Source: three-view drawing plus pictorial views. Frame: mm from the lowest corner of the part. A direction names the side the tool comes from. Round coordinates to 2 decimals unless told otherwise and drop trailing zeros. Order: outer loops, then holes, each group sorted by start corner. A loop starts at its lowest first (then second) coordinate and runs counter-clockwise, first axis right, second up. Notation, with made-up numbers: (-29.5, -19.75) -> (19.5, -19.75) arc R6 ccw to (19.5, -14.75) -> close; hole circle Ø10 at (4.5, 64). An arc over 180 degrees is marked (long way). Answer as CSV lines item,"result". Start each with the question number.
1) First-contact query: P1, Ø0.6, axis at x = 15, y = 22, coming from the -Z side; P2, Ø12, axis at x = 16, z = 18.5, coming from the +Y side; P3, Ø7, axis at x = 47.5, y = 18.5, coming from the +Z side. Flat tips, straight axial feed; report the tip coordinate or a pass-through.
2) Access query for the marked faces 4 and 5. Directions: +Z, -Z, +X, -X, +Y, -Y. A direction counts if a zero-diameter tool reaches every point of the face in a straight line with its end or side. Return the directions, or none.
3) Section query B-B, the plane x = 14.5. Output: boundary loops of the cut face in (y, z).
4) Mould query, pull axis Z, two halves, no side actions, for the marked faces 1, 2 and 3. Classes: +Z half, -Z half, draft (parallel to the pull), parting line (faces both ways), or undercut.
5) Section query C-C, the plane y = 4. Output: boundary loops of the cut face in (x, z), and give its area (3 significant figures).
6) Section query A-A, the plane z = 33. Output: boundary loops of the cut face in (x, y), and give its area (3 significant figures).
7) Section query D-D, the plane z = 40.5. Output: boundary loops of the cut face in (x, y).
8) Line query: L1, parallel to Y at x = 33, z = 39.5; L2, parallel to Z at x = 34.5, y = 11.5; L3, parallel to Y at x = 17, z = 25. Output: solid intervals per line, ascending.
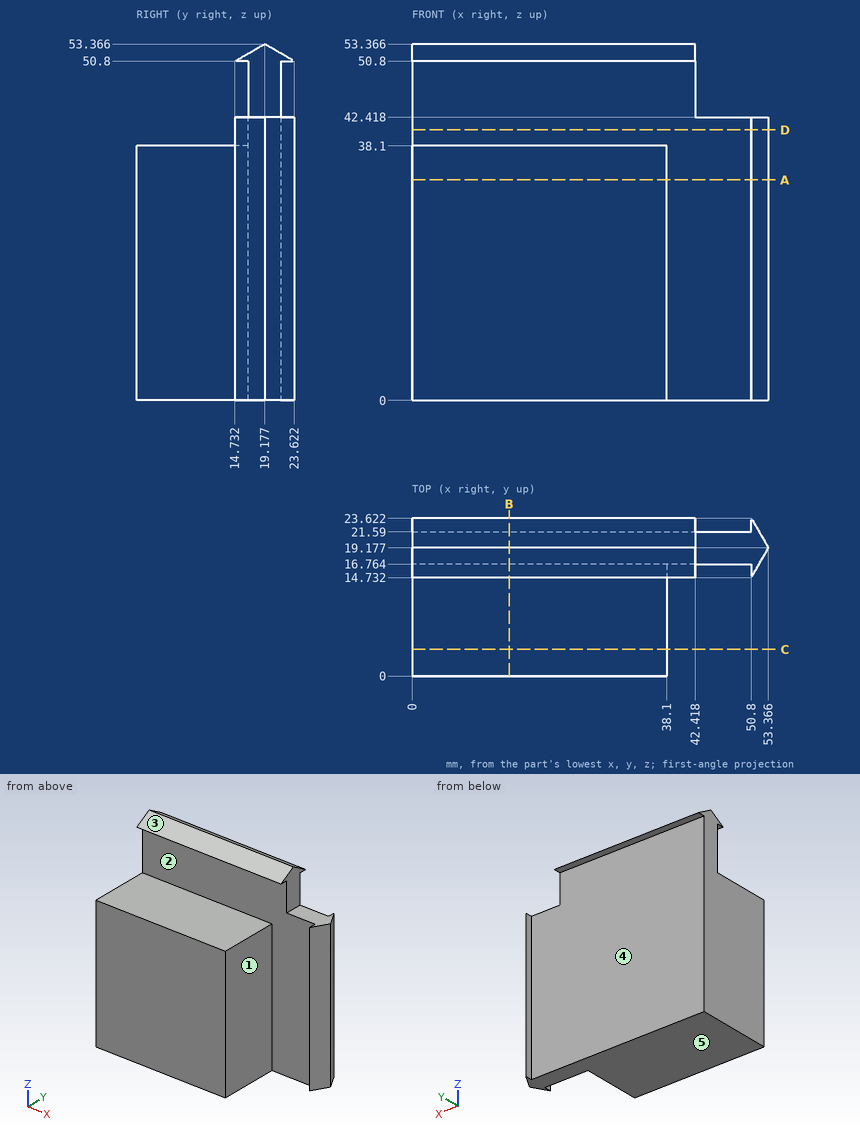
Findings:
1,P1,"stops at z = 50.8"
1,P2,"stops at y = 21.59"
1,P3,"stops at z = 42.42"
2,face 4,"-Z, -X, +Y"
2,face 5,"-Z, +X, -X, +Y, -Y"
3,outline,"(0, 0) -> (21.59, 0) -> (21.59, 50.8) -> (23.62, 50.8) -> (19.18, 53.37) -> (14.73, 50.8) -> (16.76, 50.8) -> (16.76, 38.1) -> (0, 38.1) -> close"
4,face 1,"draft"
4,face 2,"undercut"
4,face 3,"+Z half"
5,outline,"(0, 0) -> (38.1, 0) -> (38.1, 38.1) -> (0, 38.1) -> close"
5,area,"1,450 mm^2"
6,outline,"(0, 0) -> (38.1, 0) -> (38.1, 16.76) -> (50.8, 16.76) -> (50.8, 14.73) -> (53.37, 19.18) -> (50.8, 23.62) -> (50.8, 21.59) -> (0, 21.59) -> close"
6,area,"895 mm^2"
7,outline,"(0, 16.76) -> (50.8, 16.76) -> (50.8, 14.73) -> (53.37, 19.18) -> (50.8, 23.62) -> (50.8, 21.59) -> (0, 21.59) -> close"
8,L1,"y = 16.76 to 21.59"
8,L2,"z = 0 to 38.1"
8,L3,"y = 0 to 21.59"
